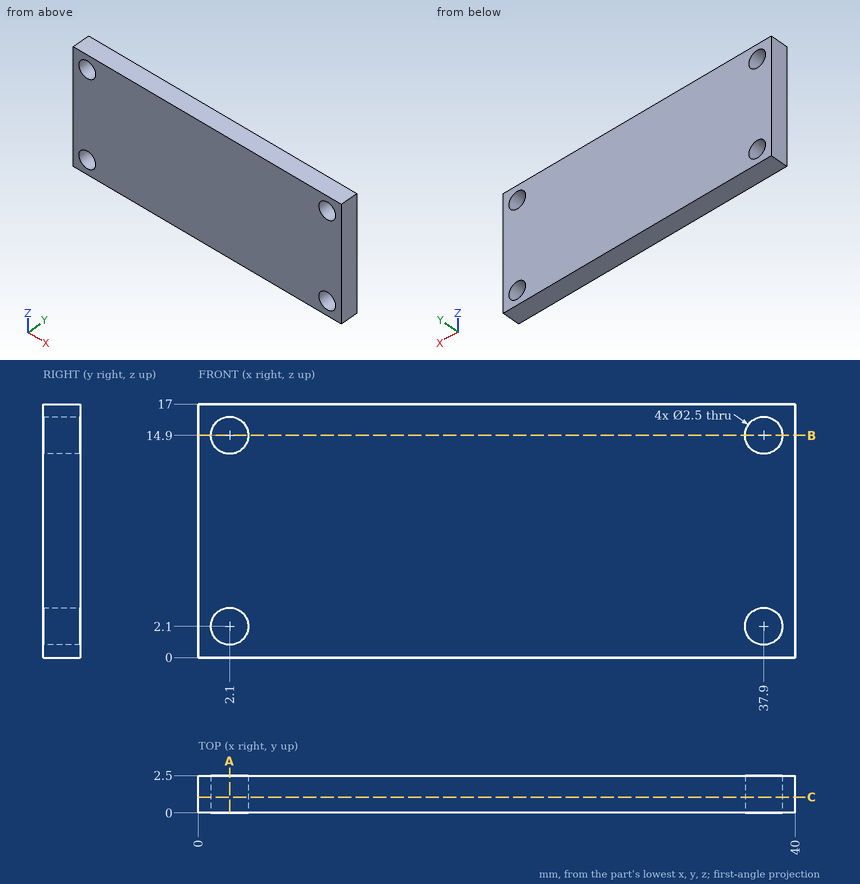
Answer from the drawing. Dimensions are ordinates in mm from the lowest x, y and z of the part. Coordinates: 2 decimals unless noted, no trailing zeros. Order: outer loops, then holes, each group sorted by start corner. A loop starts at its lowest first (then second) coordinate and runs counter-clockwise, first axis right, second up. Notation, with made-up numbers: (-3.5, -38) - (35.5, -38) arc R28 ccw to (35.5, -16) - close; hole circle Ø10 at (-1.5, 76.25). An arc over 180 degrees is marked (long way). Put each result on its own line as item: value. Start each with the question number.
1) Find section A-A (x = 2.1). Give the vertices of the cut face in (y, z).
2) Find the intervals of material crossed by line 1 (Z direction, x = 38, y = 1.35); line 2 (X direction, y = 0.9, z = 2.1); line 3 (X direction, y = 0.15, z = 1.5), in increasing order. Write a range as from..to.
3) Find section C-C (y = 1.05). Give the vertices of the cut face in (x, z).
4) Find section B-B (z = 14.9). Give the vertices of the cut face in (x, y), plus the area to 3 significant figures.
Results list:
1. outline: (0, 0) - (2.5, 0) - (2.5, 0.85) - (0, 0.85) - close; (0, 3.35) - (2.5, 3.35) - (2.5, 13.65) - (0, 13.65) - close; (0, 16.15) - (2.5, 16.15) - (2.5, 17) - (0, 17) - close
2. line 1: z = 0..0.85, 3.35..13.65, 16.15..17
2. line 2: x = 0..0.85, 3.35..36.65, 39.15..40
2. line 3: x = 0..1, 3.2..36.8, 39..40
3. outline: (0, 0) - (40, 0) - (40, 17) - (0, 17) - close; hole circle Ø2.5 at (2.1, 2.1); hole circle Ø2.5 at (2.1, 14.9); hole circle Ø2.5 at (37.9, 2.1); hole circle Ø2.5 at (37.9, 14.9)
4. outline: (0, 0) - (0.85, 0) - (0.85, 2.5) - (0, 2.5) - close; (3.35, 0) - (36.65, 0) - (36.65, 2.5) - (3.35, 2.5) - close; (39.15, 0) - (40, 0) - (40, 2.5) - (39.15, 2.5) - close
4. area: 87.5 mm^2
